```python
from build123d import *

# Parameters (mm, degrees)
SKETCH2_W           = 10
SKETCH2_H           = 10
BOSS_EXTRUDE1_DEPTH = 158.8
SKETCH3_R           = 3.5
BOSS_EXTRUDE2_DEPTH = 8
SKETCH4_W           = 15
SKETCH4_H           = 27.94
BOSS_EXTRUDE4_DEPTH = 4
SKETCH5_W           = 2.25448465
SKETCH5_H           = 27.94
BOSS_EXTRUDE5_DEPTH = 4
SKETCH6_R           = 1.5
CUT_EXTRUDE1_DEPTH  = 40
SKETCH7_W           = 15
SKETCH7_H           = 27.94
CUT_EXTRUDE2_DEPTH  = 8


with BuildPart() as part:
    # Sketch2 → Boss-Extrude1 (new body)
    with BuildSketch(Plane.XY):
        with Locations((5, 5)):
            Rectangle(SKETCH2_W, SKETCH2_H)
    extrude(amount=BOSS_EXTRUDE1_DEPTH)

    # Sketch3 → Boss-Extrude2 (add)
    with BuildSketch(Plane(origin=(10, 0, 0), x_dir=(0, 0, -1), z_dir=(1, 0, 0))):
        with Locations((-5, 5)):
            Circle(SKETCH3_R)
    extrude(amount=BOSS_EXTRUDE2_DEPTH)

    # Sketch4 → Boss-Extrude4 (add)
    with BuildSketch(Plane.XY.offset(158.8)):
        with Locations((7.5, 5)):
            Rectangle(SKETCH4_W, SKETCH4_H)
    extrude(amount=BOSS_EXTRUDE4_DEPTH)

    # Sketch5 → Boss-Extrude5 (add)
    with BuildSketch(Plane.XY.offset(162.8)):
        with Locations((13.872757675, 5)):
            Rectangle(SKETCH5_W, SKETCH5_H)
    extrude(amount=BOSS_EXTRUDE5_DEPTH)

    # Sketch6 → Cut-Extrude1 (cut)
    with BuildSketch(Plane.ZY.offset(-12.74551535)):
        with Locations((165.086, 16.64426)):
            Circle(SKETCH6_R)
        with Locations((165.086, -6.645)):
            Circle(SKETCH6_R)
    extrude(amount=-CUT_EXTRUDE1_DEPTH, mode=Mode.SUBTRACT)

    # Sketch7 → Cut-Extrude2 (cut)
    with BuildSketch(Plane.XY.offset(166.8)):
        with Locations((7.5, 5)):
            Rectangle(SKETCH7_W, SKETCH7_H)
    extrude(amount=-CUT_EXTRUDE2_DEPTH, mode=Mode.SUBTRACT)


solid = part.part
```
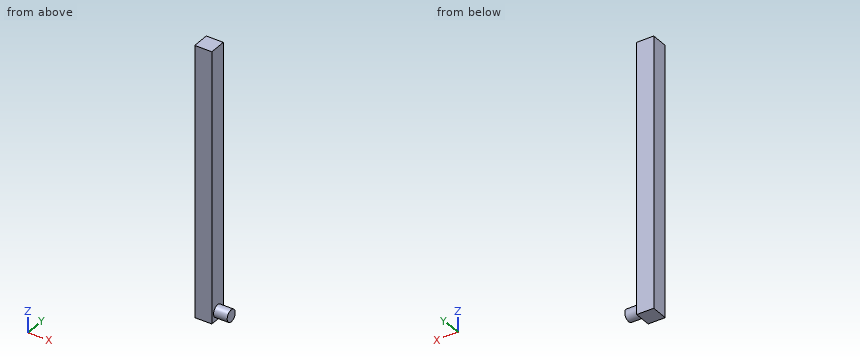
Design review of the part built by this model. Coordinates are the model's own, in mm. Round coordinates to 2 decimals unless told otherwise and drop trailing zeros. Order: outer loops, then holes, each group sorted by start corner. A loop starts at its lowest first (then second) coordinate and runs counter-clockwise, first axis right, second up. Notation, with made-up numbers: (-36, 28) - (-24, 28) arc R19 ccw to (-24, 34) - close; hole circle Ø10 at (12, 63). An arc over 180 degrees is marked (long way). Return JSON: item names as keys, results as strings.
Q1. Wall thickness on L1, parallel to X at y = 2.5, z = 107.5; L2, parallel to Z at x = 15.75, y = 7.75; L3, parallel to Z at x = 12.5, y = 3: over which ranges is each line inside the solid? List them lowest first. Write a range as [from, to].
Computed values:
{"L1": "x = [0, 10]", "L2": "z = [2.83, 7.17]", "L3": "z = [2.13, 7.87]"}
Q2. Consider section B-B on z = 5. Write out the cut boundary in (x, y), plus the area to 3 significant figures.
Computed values:
{"outline": "(0, 0) - (10, 0) - (10, 1.5) - (18, 1.5) - (18, 8.5) - (10, 8.5) - (10, 10) - (0, 10) - close", "area": "156 mm2"}
Q3. Consider section A-A on y = 5. Write out the cut boundary in (x, z), plus the area to 3 significant figures.
Computed values:
{"outline": "(0, 0) - (10, 0) - (10, 1.5) - (18, 1.5) - (18, 8.5) - (10, 8.5) - (10, 158.8) - (0, 158.8) - close", "area": "1,640 mm2"}
Q4. For pin 1 Ø10 at (x, z) = (5, 49.5) entering from -Y; pin 2 Ø1 at (x, y) = (12.5, 3.5) entering from -Z; pin 3 Ø2 at (x, y) = (13.5, 1.5) entering from -Z, all flat-tipped, find the tip position at first contact; note any pin that passes through.
Computed values:
{"pin 1": "stops at y = 0", "pin 2": "stops at z = 1.65", "pin 3": "stops at z = 2.55"}
Q5. Consider section C-C on x = 14.75. Write out the cut boundary in (y, z).
Computed values:
{"outline": "circle Ø7 at (5, 5)"}
